from build123d import *

# Parameters (mm, degrees)
SKETCH_W        = 10.8
SKETCH_H        = 10.8
PAD_DEPTH       = 10.8
THICKNESS_T     = 1
SKETCH001_W     = 10.8
SKETCH001_H     = 1
PAD001_DEPTH    = 6
SKETCH002_R     = 1.4
POCKET_DEPTH    = 1.001
SKETCH003_W     = 6
SKETCH003_H     = 3.3
POCKET001_DEPTH = 5
SKETCH004_W     = 4.8
SKETCH004_H     = 4.8
POCKET002_DEPTH = 1
SKETCH005_W     = 4.8
SKETCH005_H     = 4.8
POCKET003_DEPTH = 12.801


with BuildPart() as part:
    # Sketch → Pad (new body)
    with BuildSketch(Plane.XY):
        with Locations((5.4, 5.4)):
            Rectangle(SKETCH_W, SKETCH_H)
    extrude(amount=PAD_DEPTH)

    # Thickness
    thickness_openings = [part.faces().sort_by_distance(p)[0] for p in [
        (5.4, 5.4, 10.8),
    ]]
    offset(amount=THICKNESS_T, openings=thickness_openings)

    # Sketch001 → Pad001 (new body)
    with BuildSketch(Plane.XY.offset(10.8)):
        with Locations((5.4, 11.3)):
            Rectangle(SKETCH001_W, SKETCH001_H)
    extrude(amount=PAD001_DEPTH)

    # Sketch002 → Pocket (cut, through all)
    with BuildSketch(Plane.XZ.offset(-10.8)):
        with Locations((5.4, 13.8)):
            Circle(SKETCH002_R)
    extrude(amount=-POCKET_DEPTH, mode=Mode.SUBTRACT)

    # Sketch003 → Pocket001 (cut)
    with BuildSketch(Plane.XY):
        with Locations((5.4, 9.15)):
            Rectangle(SKETCH003_W, SKETCH003_H)
    extrude(amount=-POCKET001_DEPTH, mode=Mode.SUBTRACT)

    # Sketch004 → Pocket002 (cut)
    with BuildSketch(Plane.XZ.offset(1)):
        with Locations((5.4, 5.4)):
            Rectangle(SKETCH004_W, SKETCH004_H)
    extrude(amount=-POCKET002_DEPTH, mode=Mode.SUBTRACT)

    # Sketch005 → Pocket003 (cut, through all)
    with BuildSketch(Plane.YZ.offset(11.8)):
        with Locations((5.4, 5.4)):
            Rectangle(SKETCH005_W, SKETCH005_H)
    extrude(amount=-POCKET003_DEPTH, mode=Mode.SUBTRACT)


solid = part.part
Can you work these out from the model? Positions are in its coordinate system, mm. A direction names the side the tool comes from. Coordinates: 2 decimals unless noted, no trailing zeros. Loops run counter-clockwise (first coordinate to the right, second up) from the corner with the lowest first, then second, coordinate; pieces in that order, holes last. Notation, with made-up numbers: (14.5, 6) - (57.5, 6) arc R18 cw to (57.5, 33) - close; hole circle Ø11 at (81.25, 39.5). An arc over 180 degrees is marked (long way). Put each result on its own line as item: value. Start each with the question number.
Item 1: Suppose I cut it at D-D (z = 13.8). Please give me the cut outline in (x, y).
Item 2: Suppose I cut it at C-C (y = 9.5). Please give me the cut outline in (x, z).
Item 3: If I drill on line 1 along X through (y, z) = (2.75, 5.75); line 2 along Z through (x, y) = (3, 2), over which ranges is the centre line in solid material (lowest first)?
Item 4: Suppose I cut it at B-B (x = 3.75). Please give me the cut outline in (y, z), and give its area (3 significant figures).
Item 5: For pin 1 (0.5 mm diameter, centred on x = -0.5, z = 5.5, fed in from +Y); pin 2 (1.1 mm diameter, centred on x = 11.5, z = 6.5, fed in from -Y); pin 3 (1.7 mm diameter, centred on x = 5.4, z = 13.8, fed in from +Y); pin 4 (0.8 mm diameter, centred on x = 5.5, y = -0.5, fed in from -Z) (3 decimals), each with a flat end and sliding along its axis, tell me the tip position at first contact or that it passes through.
Item 6: Suppose I cut it at A-A (y = 5). Please give me the cut outline in (x, z).
Item 7: If we mould it in two halves opening along Y, with no side actions, what happens to faces 1 (the face through (11.499, -0.715, 5.476)), 2 (the face through (-0.5, 5.4, 3)), 3 (the face through (2.4, 9.1, -0.5)), 4 (the face through (5, 11.8, 8))? For each: +Y half, -Y half, draft (parallel to the pull), parting line (faces both ways), or undercut.
Item 8: Which directions (+Z, -Z, +X, -X, +Y, -Y) give clear straight access to the entire face, cutting with the end or side of a thin tool? Please do faces 5 (the face through (3, -0.5, 5.4)), 6 (the face through (-0.5, 3, 5.4)), 7 (the face through (0, 11, 14)).
Here are the results:
1. outline: (0, 10.8) - (4, 10.8) - (4, 11.8) - (0, 11.8) - close; (6.8, 10.8) - (10.8, 10.8) - (10.8, 11.8) - (6.8, 11.8) - close
2. outline: (-1, 0) arc R1 ccw to (0, -1) - (2.4, -1) - (2.4, 0) - (0, 0) - (0, 10.8) - (-1, 10.8) - close; (8.4, -1) - (10.8, -1) arc R1 ccw to (11.8, 0) - (11.8, 10.8) - (10.8, 10.8) - (10.8, 0) - (8.4, 0) - close
3. line 1: -1 to 0, 10.8 to 11.8
3. line 2: -1 to 0
4. outline: (-1, 0) arc R1 ccw to (0, -1) - (7.5, -1) - (7.5, 0) - (0, 0) - (0, 3) - (-1, 3) - close; (-1, 7.8) - (0, 7.8) - (0, 10.8) - (-1, 10.8) - close; (10.8, -1) arc R1 ccw to (11.8, 0) - (11.8, 16.8) - (10.8, 16.8) - close
4. area: 31.9 mm²
5. pin 1: y = 11.77
5. pin 2: y = -0.99
5. pin 3: through
5. pin 4: z = -0.995
6. outline: (-1, 0) arc R1 ccw to (0, -1) - (10.8, -1) arc R1 ccw to (11.8, 0) - (11.8, 3) - (10.8, 3) - (10.8, 0) - (0, 0) - (0, 3) - (-1, 3) - close; (-1, 7.8) - (0, 7.8) - (0, 10.8) - (-1, 10.8) - close; (10.8, 7.8) - (11.8, 7.8) - (11.8, 10.8) - (10.8, 10.8) - close
7. face 1: -Y half
7. face 2: undercut
7. face 3: undercut
7. face 4: +Y half
8. face 5: -Y
8. face 6: +X, -X
8. face 7: +Z, -X, +Y, -Y
